```python
from build123d import *

# Parameters (mm, degrees)
F1_DEPTH = 63.5
F2_DEPTH = 25.4
F3_DEPTH = 7.9375
F0_W     = 25.5907994721
F0_H     = 19.05
F5_R     = 6.35


with BuildPart() as f1:
    # F0 (on Front) → F1 (new body, symmetric)
    with BuildSketch(Plane.XZ):
        Polygon((22.225, 9.525), (-41.275, 9.525), (-41.275, -9.525), (41.275, -9.525), (41.275, 9.525), align=None)
    extrude(amount=F1_DEPTH, both=True)

    # F0 (on Front) → F2 (join, symmetric)
    with BuildSketch(Plane.XZ):
        with BuildLine():
            Line((22.225, 27.0002), (22.225, 9.525))
            Line((22.225, 9.525), (41.275, 9.525))
            Line((41.275, 9.525), (41.275, 27.0002))
            ThreePointArc((41.275, 27.0002), (45.9246798487, 38.2255201513), (57.15, 42.8752))
            Line((57.15, 42.8752), (60.325, 42.8752))
            Line((60.325, 42.8752), (60.325, 61.9252))
            Line((60.325, 61.9252), (57.15, 61.9252))
            add(Edge.make_bspline(
                [(51.5354770489, 61.4709521971), (53.4127539881, 61.6507047986), (55.2854096398, 61.802043629), (57.15, 61.9252)],
                knots=[106.4817518013, 106.4817518013, 106.4817518013, 106.4817518013, 111.5045361635, 111.5045361635, 111.5045361635, 111.5045361635], degree=3))
            ThreePointArc((51.5354770489, 61.4709521971), (30.5432072671, 49.6239531251), (22.225, 27.0002))
        make_face()
    extrude(amount=F2_DEPTH, both=True)

    # F0 (on Front) → F3 (join, symmetric)
    with BuildSketch(Plane.XZ):
        with BuildLine():
            add(Edge.make_bspline(
                [(-41.275, 9.525), (-30.1370525235, 41.0795542305), (11.7376830989, 57.6602427342), (51.5354770489, 61.4709521971)],
                knots=[0, 0, 0, 0, 106.4817518013, 106.4817518013, 106.4817518013, 106.4817518013], degree=3))
            Line((-41.275, 9.525), (22.225, 9.525))
            Line((22.225, 9.525), (22.225, 27.0002))
            ThreePointArc((22.225, 27.0002), (30.5432072671, 49.6239531251), (51.5354770489, 61.4709521971))
        make_face()
    extrude(amount=F3_DEPTH, both=True)

    # F0 (on Front) → F4 (revolve)
    with BuildSketch(Plane.XZ):
        with Locations((73.120399736, 52.4002)):
            Rectangle(F0_W, F0_H)
    revolve(axis=Axis((60.325, 0, 52.3875), (0, 0, 1)))

    # F5
    f5_edges = [f1.edges().sort_by_distance(p)[0] for p in [
        (41.275, -63.5, 0),
        (-41.275, -63.5, 0),
        (-41.275, 63.5, 0),
        (41.275, 63.5, 0),
    ]]
    fillet(f5_edges, radius=F5_R)


solid = f1.part
```
Verification items for the finished model (mm, model axes). A direction names the side the tool comes from. Coordinates: 2 decimals unless noted, no trailing zeros. Write each loop counter-clockwise with the first axis right and the second up, starting at its lowest first coordinate (ties: lowest second). Pieces come first, ordered by that corner, then holes. Notation, with made-up numbers: M -22.5,53 L 29.5,53 A28 ccw 29.5,87 Z; hole C -3,32 d3. An arc over 180 degrees is marked long. Answer as a JSON object with one key per item and string values. Group by question number.
(1) Cross-section at B-B, the plane y = 47. Record the cut outline in (x, z) (3 decimals), and give its area (3 significant figures).
(2) Tool access check on faces 1 (the face through (41.275, -1, 4)), 2 (the face through (34.74, 0.52, 59.99)), 3 (the face through (27.52, 16.55, 45.49)), 4 (the face through (22.225, -17, 18)). Record the directions out of +Z, -Z, +X, -X, +Y, -Y that give a thin tool (end or side, any length) a straight path to the whole face; none if there is none.
(3) Cross-section at C-C, the plane x = 77.5. Record the cut outline in (y, z).
(4) Cross-section at A-A, the plane z = 6. Record the cut outline in (x, y) (3 decimals), and give its area (3 significant figures).
(5) Material ranges on line 1 (Z direction, x = 10, y = 12) (3 decimals); line 2 (Y direction, x = 39, z = 24); line 3 (X direction, y = -45, z = -6) (3 decimals), recorded low to high.
(6) Gauge pin test, flat ends, axial feed: pin 1 (1.5 mm diameter, centred on y = -31.5, z = 4.5, fed in from +X) (3 decimals); pin 2 (23 mm diameter, centred on x = 69.5, y = 7, fed in from -Z); pin 3 (25 mm diameter, centred on x = 3.5, z = 27, fed in from +Y). Record the tip position at first contact, or that the pin passes through.
Reply:
{
 "1": {"outline": "M -41.275,-9.525 L 41.275,-9.525 L 41.275,9.525 L -41.275,9.525 Z", "area": "1,570 mm²"},
 "2": {"face 1": "-Z, +X, +Y, -Y", "face 2": "+Z, -X", "face 3": "+Z, -X, +Y", "face 4": "+Z, -X, -Y"},
 "3": {"outline": "M -18.97,42.88 L 18.97,42.88 L 18.97,61.93 L -18.97,61.93 Z"},
 "4": {"outline": "M -41.275,-57.15 A6.35 ccw -34.925,-63.5 L 34.925,-63.5 A6.35 ccw 41.275,-57.15 L 41.275,57.15 A6.35 ccw 34.925,63.5 L -34.925,63.5 A6.35 ccw -41.275,57.15 Z", "area": "10,400 mm²"},
 "5": {"line 1": "-9.525 to 9.525", "line 2": "-25.4 to 25.4", "line 3": "-41.275 to 41.275"},
 "6": {"pin 1": "x = 41.275", "pin 2": "z = 42.88", "pin 3": "y = 7.94"}
}
